The drawing under review shows one solid part. Ordinate dimensions are in mm from its lowest x, y, z. Give positions to 0.01 mm unless a question says otherwise; leave off trailing zeros. Order: outer loops, then holes, each group sorted by start corner. A loop starts at its lowest first (then second) coordinate and runs counter-clockwise, first axis right, second up. Notation, with made-up numbers: (11, -24.5) -> (27, -24.5) arc R16 cw to (27, -4.5) -> close; hole circle Ø10 at (-35.75, -32). An arc over 180 degrees is marked (long way). Return JSON: item names as keys, results as strings. Group by question number.
1) Add section C-C (x = 15.25). Give the boundary of the cut face in (y, z).
2) Add section B-B (z = 2.55). State how many separate pieces and enclosed holes the cut face has, then the cut area to 3 significant figures.
3) Add section A-A (y = 123). Give the boundary of the cut face in (x, z), then the cut area to 3 significant figures.
4) To check wall thickness, follow line 1 along X through (y, z) = (88.25, 3.1); line 2 along Y through (x, z) = (40, 3.55); line 3 along X through (y, z) = (86.5, 4.4). State the ranges of each line that lie inside material, in increasing order.
5) Insertion check: P1, Ø4, axis at x = 64.75, y = 137.75, coming from the +Z side; P2, Ø1.5, axis at x = 29, z = 4, coming from the -Y side. Each pin has a flat end and moves straight along its axis. Give the tip position at first contact, or say it passes through.
6) Add section D-D (y = 14.5). Give the boundary of the cut face in (x, z).
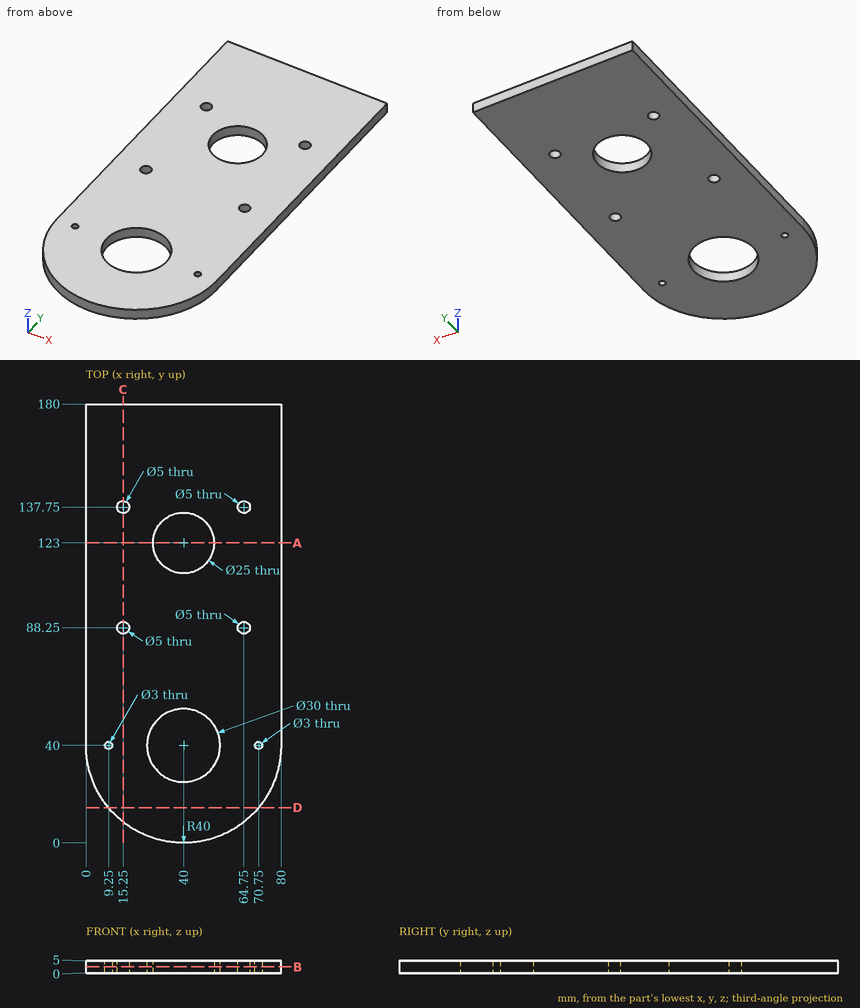
Evaluation:
{
 "1": {"outline": "(8.58, 0) -> (85.75, 0) -> (85.75, 5) -> (8.58, 5) -> close; (90.75, 0) -> (135.25, 0) -> (135.25, 5) -> (90.75, 5) -> close; (140.25, 0) -> (180, 0) -> (180, 5) -> (140.25, 5) -> close"},
 "2": {"separate pieces": "1", "enclosed holes": "8", "area": "12,400 mm^2"},
 "3": {"outline": "(0, 0) -> (27.5, 0) -> (27.5, 5) -> (0, 5) -> close; (52.5, 0) -> (80, 0) -> (80, 5) -> (52.5, 5) -> close", "area": "275 mm^2"},
 "4": {"line 1": "0 to 12.75, 17.75 to 62.25, 67.25 to 80", "line 2": "0 to 25, 55 to 110.5, 135.5 to 180", "line 3": "0 to 13.46, 17.04 to 62.96, 66.54 to 80"},
 "5": {"P1": "through", "P2": "y = 1.34"},
 "6": {"outline": "(9.18, 0) -> (70.82, 0) -> (70.82, 5) -> (9.18, 5) -> close"}
}
